The figure shows three views and two pictorial views of one solid part (mm, origin at its lowest corner). Answer the questions. Coordinates: 2 decimals unless noted, no trailing zeros. Order: outer loops, then holes, each group sorted by start corner. A loop starts at its lowest first (then second) coordinate and runs counter-clockwise, first axis right, second up. Notation, with made-up numbers: (-22, 86) -> (-4, 86) arc R18 ccw to (-4, 103) -> close; hole circle Ø11 at (-25.75, -29). An arc over 180 degrees is marked (long way). Return JSON: item names as keys, results as strings. Group by question number.
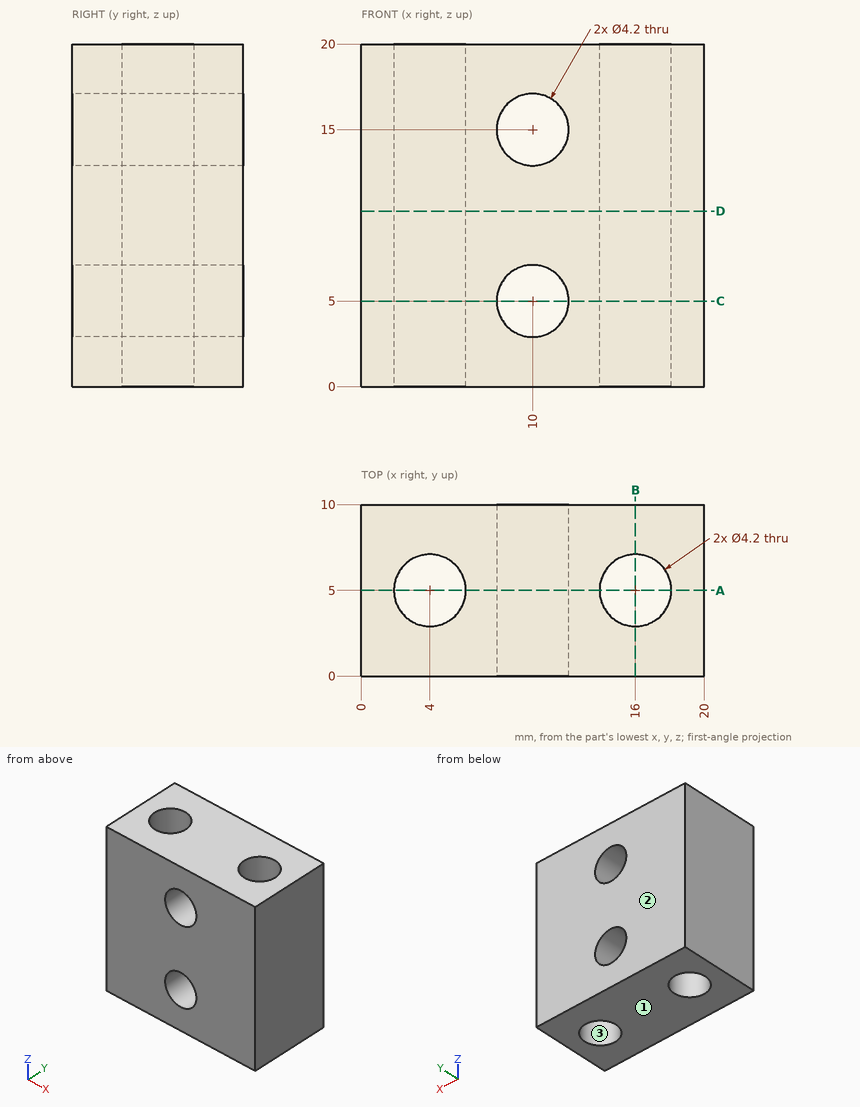
1. Find section C-C on z = 5. Determine the outline of the cut face in (x, y), and give its area (3 significant figures).
2. Straight lines are drawn through the part: L1, parallel to Z at x = 10, y = 7.75; L2, parallel to Y at x = 16, z = 5.75; L3, parallel to Z at x = 11.75, y = 1.25. For each, find the intervals that lie inside material, in ascending order.
3. Find section A-A on y = 5. Determine the outline of the cut face in (x, z).
4. Find section D-D on z = 10.25. Determine the outline of the cut face in (x, y), and give its area (3 significant figures).
5. Find section B-B on x = 16. Determine the outline of the cut face in (y, z), and give its area (3 significant figures).
6. For a pull along Y with two mould halves and no side action, classify the marked faces 1, 2 and 3 as released by +Y, released by -Y, zero draft, split by the parting line, or undercut.
Result:
{
 "1": {"outline": "(0, 0) -> (7.9, 0) -> (7.9, 10) -> (0, 10) -> close; (12.1, 0) -> (20, 0) -> (20, 10) -> (12.1, 10) -> close; hole circle Ø4.2 at (4, 5); hole circle Ø4.2 at (16, 5)", "area": "130 mm^2"},
 "2": {"L1": "0 to 2.9, 7.1 to 12.9, 17.1 to 20", "L2": "0 to 2.9, 7.1 to 10", "L3": "0 to 3.84, 6.16 to 13.84, 16.16 to 20"},
 "3": {"outline": "(0, 0) -> (1.9, 0) -> (1.9, 20) -> (0, 20) -> close; (6.1, 0) -> (13.9, 0) -> (13.9, 20) -> (6.1, 20) -> close; (18.1, 0) -> (20, 0) -> (20, 20) -> (18.1, 20) -> close; hole circle Ø4.2 at (10, 5); hole circle Ø4.2 at (10, 15)"},
 "4": {"outline": "(0, 0) -> (20, 0) -> (20, 10) -> (0, 10) -> close; hole circle Ø4.2 at (4, 5); hole circle Ø4.2 at (16, 5)", "area": "172 mm^2"},
 "5": {"outline": "(0, 0) -> (2.9, 0) -> (2.9, 20) -> (0, 20) -> close; (7.1, 0) -> (10, 0) -> (10, 20) -> (7.1, 20) -> close", "area": "116 mm^2"},
 "6": {"face 1": "zero draft", "face 2": "released by +Y", "face 3": "undercut"}
}
